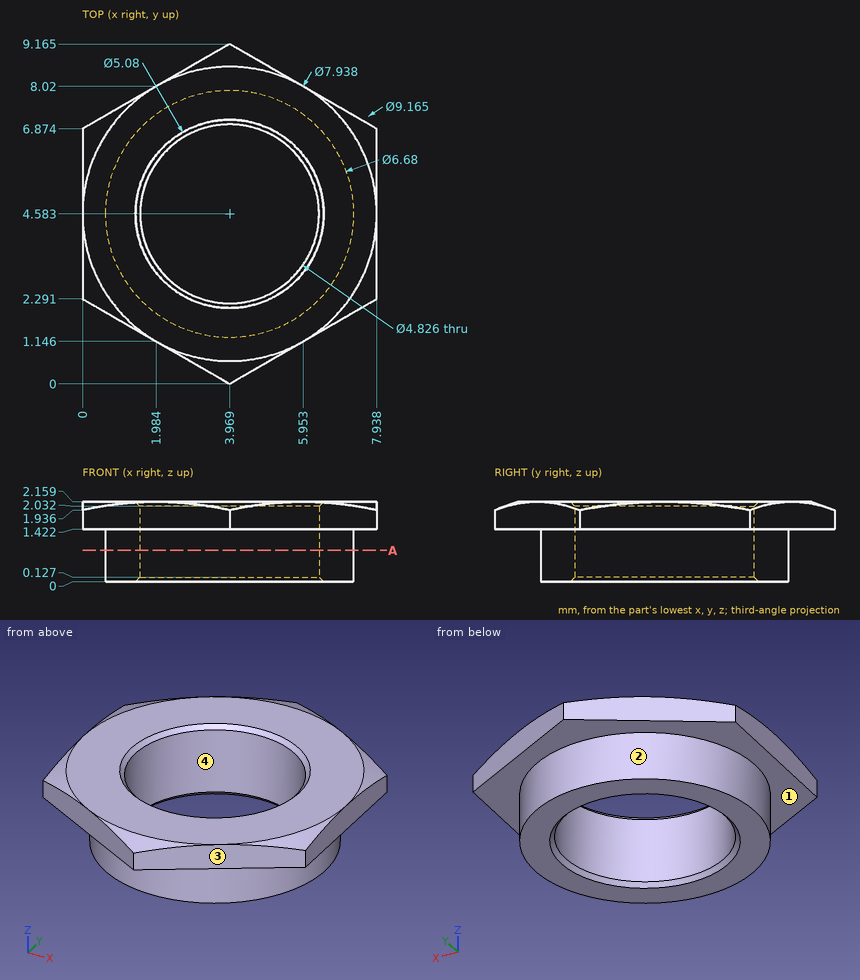
Study the drawing (mm; zero at the part's minimum x, y, z) and answer. Round coordinates to 2 decimals unless told otherwise and drop trailing zeros. Loops run counter-clockwise (first coordinate to the right, second up) from the corner with the lowest first, then second, coordinate; pieces in that order, holes last. Notation, with made-up numbers: (2, 57) - (58, 57) arc R23 ccw to (58, 95) - close; hole circle Ø11 at (-18, -10). An arc over 180 degrees is marked (long way). Use one line per item in the form item = value. Start each with the question number.
1. For a pull along Y with two mould halves and no side action, classify the marked faces 1, 2, 3 and 4 as pulls with the +Y half, pulls with the -Y half, needs draft (parallel to the pull), parting line crosses it, or undercut.
2. Consider line 1 (Z direction, x = 1, y = 2.5); line 2 (X direction, y = 3.25, z = 1.9) (1 decimal); line 3 (X direction, y = 3.25, z = 1) (1 decimal). Determine where each line is inside the solid, lowest interval first. Write a range as [from, to].
3. The part is cut by section A-A on z = 0.85. Determine the outline of the cut face in (x, y) (1 decimal).
Geometry check:
q1.face_1 = needs draft
q1.face_2 = parting line crosses it
q1.face_3 = pulls with the -Y half
q1.face_4 = undercut
q2.line_1 = [1.42, 2.16]
q2.line_2 = [0, 2], [6, 7.9]
q2.line_3 = [0.9, 2], [6, 7]
q3.outline = circle Ø6.7 at (4, 4.6); hole circle Ø4.8 at (4, 4.6)
